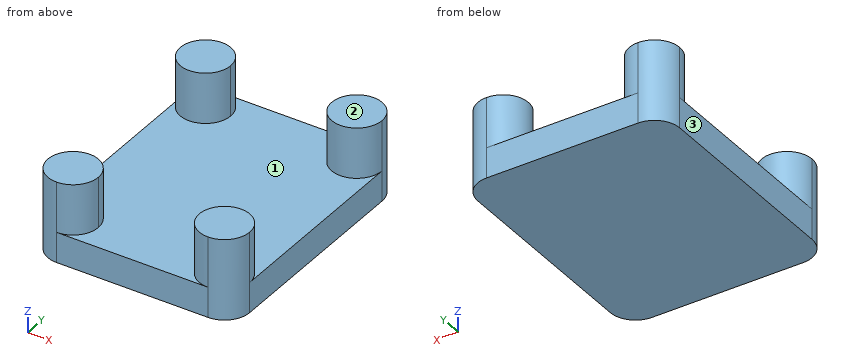
from build123d import *

# Parameters (mm, degrees)
F1_DEPTH = 3
F2_DEPTH = 5


with BuildPart() as f1:
    # F0 (on Top) → F1 (new body)
    with BuildSketch(Plane.XY):
        with BuildLine():
            ThreePointArc((-7.5, 12.5), (-5.732233, 11.767767), (-5, 10))
            ThreePointArc((-5, 10), (-7.5, 7.5), (-10, 10))
            Line((-10, 10), (-10, -10))
            ThreePointArc((-10, -10), (-7.5, -7.5), (-5, -10))
            ThreePointArc((-5, -10), (-5.732233, -11.767767), (-7.5, -12.5))
            Line((-7.5, -12.5), (7.5, -12.5))
            ThreePointArc((7.5, -12.5), (5.732233, -8.232233), (10, -10))
            Line((10, -10), (10, 10))
            ThreePointArc((10, 10), (5.732233, 8.232233), (7.5, 12.5))
            Line((7.5, 12.5), (-7.5, 12.5))
        make_face()
        with BuildLine():
            ThreePointArc((7.5, -12.5), (9.267767, -11.767767), (10, -10))
            ThreePointArc((10, -10), (5.732233, -8.232233), (7.5, -12.5))
        make_face()
        with BuildLine():
            ThreePointArc((-5, -10), (-7.5, -7.5), (-10, -10))
            ThreePointArc((-10, -10), (-9.267767, -11.767767), (-7.5, -12.5))
            ThreePointArc((-7.5, -12.5), (-5.732233, -11.767767), (-5, -10))
        make_face()
        with BuildLine():
            ThreePointArc((-10, 10), (-7.5, 7.5), (-5, 10))
            ThreePointArc((-5, 10), (-5.732233, 11.767767), (-7.5, 12.5))
            ThreePointArc((-7.5, 12.5), (-9.267767, 11.767767), (-10, 10))
        make_face()
        with BuildLine():
            ThreePointArc((10, 10), (9.267767, 11.767767), (7.5, 12.5))
            ThreePointArc((7.5, 12.5), (5.732233, 8.232233), (10, 10))
        make_face()
    extrude(amount=-F1_DEPTH)

    # F0 (on Top) → F2 (join)
    with BuildSketch(Plane.XY):
        with BuildLine():
            ThreePointArc((-5, -10), (-7.5, -7.5), (-10, -10))
            ThreePointArc((-10, -10), (-9.267767, -11.767767), (-7.5, -12.5))
            ThreePointArc((-7.5, -12.5), (-5.732233, -11.767767), (-5, -10))
        make_face()
        with BuildLine():
            ThreePointArc((7.5, -12.5), (9.267767, -11.767767), (10, -10))
            ThreePointArc((10, -10), (5.732233, -8.232233), (7.5, -12.5))
        make_face()
        with BuildLine():
            ThreePointArc((10, 10), (9.267767, 11.767767), (7.5, 12.5))
            ThreePointArc((7.5, 12.5), (5.732233, 8.232233), (10, 10))
        make_face()
        with BuildLine():
            ThreePointArc((-10, 10), (-7.5, 7.5), (-5, 10))
            ThreePointArc((-5, 10), (-5.732233, 11.767767), (-7.5, 12.5))
            ThreePointArc((-7.5, 12.5), (-9.267767, 11.767767), (-10, 10))
        make_face()
    extrude(amount=F2_DEPTH)


solid = f1.part
Verification items for the finished model (mm, model axes). Face numbers are marked on the shaded views. Give positions to 0.01 mm unless a question says otherwise; leave off trailing zeros. Loops run counter-clockwise (first coordinate to the right, second up) from the corner with the lowest first, then second, coordinate; pieces in that order, holes last.
1) Draft check along X on the marked faces 1, 2 and 3. Enter one of: pulls with the +X half, pulls with the -X half, needs draft (parallel to the pull), parting line crosses it, or undercut.
2) Sectioned sample at B-B, the plane x = -0.5. Enter the section's corners in (y, z).
3) Depth check by flat-ended pin: pin 1 Ø8 at (x, y) = (3, -5.5) entering from +Z; pin 2 Ø5 at (x, y) = (-1, -1.5) entering from +Z. Enter the tip coordinate at first touch or a pass-through.
4) Sectioned sample at C-C, the plane y = -3.25. Enter the section's corners in (x, z), then the cut area to 3 significant figures.
5) Thickness scan on line 1 along Z through (x, y) = (0.25, 1.5); line 2 along Y through (x, z) = (-7, 2); line 3 along X through (y, z) = (-9.25, 2.5). Record the ranges inside material, lowest first.
6) Sectioned sample at A-A, the plane y = 8.75. Enter the section's corners in (x, z), then the cut area to 3 significant figures.
Answers:
1. face 1: undercut
1. face 2: needs draft
1. face 3: pulls with the -X half
2. outline: (-12.5, -3) - (12.5, -3) - (12.5, 0) - (-12.5, 0) - close
3. pin 1: stops at z = 5
3. pin 2: stops at z = 0
4. outline: (-10, -3) - (10, -3) - (10, 0) - (-10, 0) - close
4. area: 60.0 mm2
5. line 1: z = -3 to 0
5. line 2: y = -12.45 to -7.55, 7.55 to 12.45
5. line 3: x = -9.88 to -5.12, 5.12 to 9.88
6. outline: (-10, -3) - (10, -3) - (10, 0) - (9.67, 0) - (9.67, 5) - (5.33, 5) - (5.33, 0) - (-5.33, 0) - (-5.33, 5) - (-9.67, 5) - (-9.67, 0) - (-10, 0) - close
6. area: 103 mm2
